Work out the finished part from the listing and answer in its coordinate system (mm). Face numbers are marked on the shaded views. A direction names the side the tool comes from. Round coordinates to 2 decimals unless told otherwise and drop trailing zeros. Write each loop counter-clockwise with the first axis right and the second up, starting at its lowest first coordinate (ties: lowest second). Pieces come first, ordered by that corner, then holes. Notation, with made-up numbers: (36.25, -33) - (45.25, -33) arc R24 cw to (45.25, -22) - close; hole circle Ø4 at (60.5, 46.5). An arc over 180 degrees is marked (long way). Write item = value, one per line. Start each with the question number.
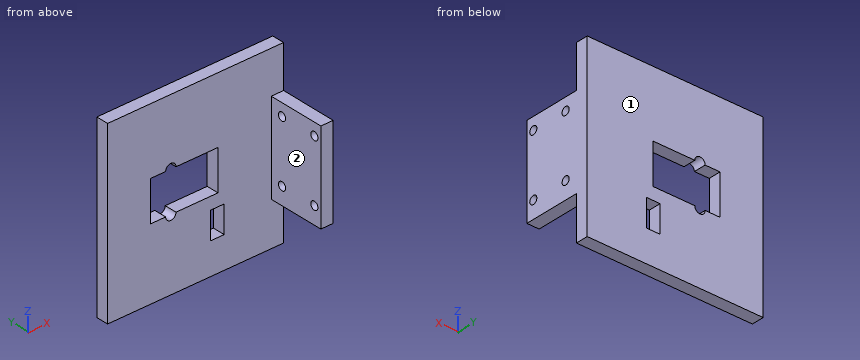
from build123d import *

# Parameters (mm, degrees)
SKETCH_1_W          = 55
SKETCH_1_H          = 70
EXTRUDE_1_DEPTH     = 5
SKETCH_2_W          = 37
SKETCH_2_H          = 28
EXTRUDE_2_DEPTH     = 5
SKETCH_3_R          = 1.65
CUT_EXTRUDE_1_DEPTH = 5
SKETCH_5_W          = 55
SKETCH_5_H          = 15.75
EXTRUDE_3_DEPTH     = 5
SKETCH_6_W          = 55
SKETCH_6_H          = 15.75
CUT_EXTRUDE_2_DEPTH = 5
CUT_EXTRUDE_3_DEPTH = 5
SKETCH_9_W          = 5.5
SKETCH_9_H          = 11
CUT_EXTRUDE_4_DEPTH = 8
SKETCH_11_W         = 16.4
SKETCH_11_H         = 70
EXTRUDE_4_DEPTH     = 5
SKETCH_12_W         = 71.4
SKETCH_12_H         = 2
EXTRUDE_5_DEPTH     = 5


with BuildPart() as part:
    # 草图1 → 凸台-拉伸1 (new body)
    with BuildSketch(Plane(origin=(0, 0, 0), x_dir=(1, 0, 0), z_dir=(0, 1, 0))):
        with Locations((27.5, -35)):
            Rectangle(SKETCH_1_W, SKETCH_1_H)
    extrude(amount=EXTRUDE_1_DEPTH)

    # 草图2 → 凸台-拉伸2 (add)
    with BuildSketch(Plane(origin=(55, 0, 0), x_dir=(0, 0, -1), z_dir=(1, 0, 0))):
        with Locations((-18.5, -9)):
            Rectangle(SKETCH_2_W, SKETCH_2_H)
    extrude(amount=-EXTRUDE_2_DEPTH)

    # 草图3 → 切除-拉伸1 (cut)
    with BuildSketch(Plane(origin=(55, 0, 0), x_dir=(0, 0, -1), z_dir=(1, 0, 0))):
        with Locations((-7, -5)):
            Circle(SKETCH_3_R)
        with Locations((-32, -5)):
            Circle(SKETCH_3_R)
        with Locations((-32, -20)):
            Circle(SKETCH_3_R)
        with Locations((-7, -20)):
            Circle(SKETCH_3_R)
    extrude(amount=-CUT_EXTRUDE_1_DEPTH, mode=Mode.SUBTRACT)

    # 草图5 → 凸台-拉伸3 (add)
    with BuildSketch(Plane(origin=(0, 5, 0), x_dir=(1, 0, 0), z_dir=(0, 1, 0))):
        with Locations((27.5, 7.875)):
            Rectangle(SKETCH_5_W, SKETCH_5_H)
    extrude(amount=-EXTRUDE_3_DEPTH)

    # 草图6 → 切除-拉伸2 (cut)
    with BuildSketch(Plane(origin=(0, 5, 0), x_dir=(1, 0, 0), z_dir=(0, 1, 0))):
        with Locations((27.5, -62.125)):
            Rectangle(SKETCH_6_W, SKETCH_6_H)
    extrude(amount=-CUT_EXTRUDE_2_DEPTH, mode=Mode.SUBTRACT)

    # 草图8 → 切除-拉伸3 (cut)
    with BuildSketch(Plane(origin=(0, 5, 0), x_dir=(1, 0, 0), z_dir=(0, 1, 0))):
        with BuildLine():
            Line((17.4, -11.1), (28.4, -11.1))
            Line((28.4, -11.1), (28.4, -27.4))
            Line((28.4, -27.4), (17.4, -27.4))
            Line((17.4, -27.4), (11.35, -27.4))
            ThreePointArc((11.35, -27.4), (9.25, -29.5), (7.15, -27.4))
            Line((7.15, -27.4), (1.1, -27.4))
            Line((1.1, -27.4), (1.1, -11.1))
            Line((1.1, -11.1), (7.15, -11.1))
            ThreePointArc((7.15, -11.1), (9.25, -9), (11.35, -11.1))
            Line((11.35, -11.1), (17.4, -11.1))
        make_face()
    extrude(amount=-CUT_EXTRUDE_3_DEPTH, mode=Mode.SUBTRACT)

    # 草图9 → 切除-拉伸4 (cut)
    with BuildSketch(Plane(origin=(0, 5, 0), x_dir=(1, 0, 0), z_dir=(0, 1, 0))):
        with Locations((28.15, -0.6)):
            Rectangle(SKETCH_9_W, SKETCH_9_H)
    extrude(amount=-CUT_EXTRUDE_4_DEPTH, mode=Mode.SUBTRACT)

    # 草图11 → 凸台-拉伸4 (add)
    with BuildSketch(Plane(origin=(0, 5, 0), x_dir=(1, 0, 0), z_dir=(0, 1, 0))):
        with Locations((-8.2, -19.25)):
            Rectangle(SKETCH_11_W, SKETCH_11_H)
    extrude(amount=-EXTRUDE_4_DEPTH)

    # 草图12 → 凸台-拉伸5 (add)
    with BuildSketch(Plane(origin=(0, 5, 0), x_dir=(1, 0, 0), z_dir=(0, 1, 0))):
        with Locations((19.3, 16.75)):
            Rectangle(SKETCH_12_W, SKETCH_12_H)
    extrude(amount=-EXTRUDE_5_DEPTH)


solid = part.part
1. Find section B-B on x = 9.25. Give the vertices of the cut face in (y, z).
2. Which of the six approach directions +Z, -Z, +X, -X, +Y, -Y give full straight-line access (tool end or side, diameter ignored) to the marked faces 1 and 2?
3. Find section A-A on z = 25. Give the vertices of the cut face in (x, y), plus the area to 4 significant figures.
4. Consider line 1 (Y direction, x = 52, z = 7); line 2 (X direction, y = 0.5, z = 6); line 3 (X direction, y = 2.75, z = 15). Determine where each line is inside the solid, lowest interval first.
5. Each of these flat-tipped pins is pushed along its axis until it touches: pin 1 (4 mm diameter, centred on x = 53.5, y = -8.5, fed in from +Z); pin 2 (5.5 mm diameter, centred on y = -5, z = 32, fed in from -X); pin 3 (10 mm diameter, centred on x = 41.5, y = -9, fed in from -Z); pin 4 (2.5 mm diameter, centred on x = 53, y = -11, fed in from -Z). Where does it stop, or does it pass through?
6. Find section D-D on x = 23.5. Give the vertices of the cut face in (y, z).
7. Find section C-C on z = 7. Give the vertices of the cut face in (x, y).
Answer key:
q1.outline = (0, -17.75) - (5, -17.75) - (5, 9) - (0, 9) - close; (0, 29.5) - (5, 29.5) - (5, 54.25) - (0, 54.25) - close
q2.face_1 = +Z, -Z, +X, -X, +Y
q2.face_2 = +Z, -Z, -X, -Y
q3.outline = (-16.4, 0) - (1.1, 0) - (1.1, 5) - (-16.4, 5) - close; (28.4, 0) - (50, 0) - (50, -23) - (55, -23) - (55, 5) - (28.4, 5) - close
q3.area = 335.5 mm²
q4.line_1 = -23 to -21.65, -18.35 to -6.65, -3.35 to 5
q4.line_2 = -16.4 to 25.4, 30.9 to 55
q4.line_3 = -16.4 to 1.1, 28.4 to 55
q5.pin_1 = 37
q5.pin_2 = 50
q5.pin_3 = through
q5.pin_4 = 0
q6.outline = (0, -17.75) - (5, -17.75) - (5, 11.1) - (0, 11.1) - close; (0, 27.4) - (5, 27.4) - (5, 54.25) - (0, 54.25) - close
q7.outline = (-16.4, 0) - (50, 0) - (50, -3.35) - (55, -3.35) - (55, 5) - (-16.4, 5) - close; (50, -23) - (55, -23) - (55, -21.65) - (50, -21.65) - close; (50, -18.35) - (55, -18.35) - (55, -6.65) - (50, -6.65) - close
